Read the model definition and answer for the solid it produces. Units are mm, in the model's axes. A direction names the side the tool comes from. Coordinates: 2 decimals unless noted, no trailing zeros. Write each loop counter-clockwise with the first axis right and the second up, starting at its lowest first coordinate (ties: lowest second). Pieces come first, ordered by that corner, then holes. Notation, with made-up numbers: (59, -36.5) -> (69, -36.5) arc R28 cw to (69, -16.5) -> close; hole circle Ø7 at (42.25, 44.25). An arc over 180 degrees is marked (long way). Return JSON: item names as keys, results as strings.
from build123d import *

# Parameters (mm, degrees)
SKETCH1_R           = 2.286
SKETCH1_R_2         = 11.1125
BOSS_EXTRUDE1_DEPTH = 16.51
SKETCH2_R           = 12.7
CUT_EXTRUDE1_DEPTH  = 1.778
FILLET1_R           = 2.54


with BuildPart() as part:
    # Sketch1 → Boss-Extrude1 (new body)
    with BuildSketch(Plane(origin=(0, 0, 0), x_dir=(0, 0, -1), z_dir=(1, 0, 0))):
        with BuildLine():
            Line((-38.739778242, 0.742722084), (-14.609778242, -80.537277916))
            ThreePointArc((-14.609778242, -80.537277916), (3.522565818, -91.027310277), (14.999447267, -73.502930908))
            Line((14.999447267, -73.502930908), (6.35, -25.4))
            Line((6.35, -25.4), (6.35, 31.75))
            Line((6.35, 31.75), (-6.35, 31.75))
            Line((-6.35, 31.75), (-31.266140037, 18.54599812))
            ThreePointArc((-31.266140037, 18.54599812), (-38.182060342, 10.978915167), (-38.739778242, 0.742722084))
        make_face()
        Circle(SKETCH1_R, mode=Mode.SUBTRACT)
        with Locations((0, 25.4)):
            Circle(SKETCH1_R, mode=Mode.SUBTRACT)
        with Locations((0, -76.2)):
            Circle(SKETCH1_R_2, mode=Mode.SUBTRACT)
        with Locations((-24.13, 5.08)):
            Circle(SKETCH1_R_2, mode=Mode.SUBTRACT)
    extrude(amount=BOSS_EXTRUDE1_DEPTH)

    # Sketch2 → Cut-Extrude1 (cut)
    with BuildSketch(Plane(origin=(16.51, 0, 0), x_dir=(0, 0, -1), z_dir=(1, 0, 0))):
        with Locations((0, -76.2)):
            Circle(SKETCH2_R)
        with Locations((-24.13, 5.08)):
            Circle(SKETCH2_R)
    extrude(amount=-CUT_EXTRUDE1_DEPTH, mode=Mode.SUBTRACT)

    # Fillet1
    fillet1_edges = [part.edges().sort_by_distance(p)[0] for p in [
        (8.255, 31.75, 6.35),
        (8.255, 31.75, -6.35),
        (8.255, -25.4, -6.35),
    ]]
    fillet(fillet1_edges, radius=FILLET1_R)


solid = part.part
1. The part is cut by section D-D (z = 27). Determine the outline of the cut face in (x, y).
Taken from the geometry:
{"outline": "(0, -38.8) -> (16.51, -38.8) -> (16.51, -7.29) -> (14.73, -7.29) -> (14.73, -5.66) -> (0, -5.66) -> close; (0, 15.82) -> (14.73, 15.82) -> (14.73, 17.45) -> (16.51, 17.45) -> (16.51, 20.81) -> (0, 20.81) -> close"}
2. The part is cut by section B-B (y = 5.08). Determine the outline of the cut face in (x, z), then the cut area to 3 significant figures.
Taken from the geometry:
{"outline": "(0, -6.35) -> (16.51, -6.35) -> (16.51, 11.43) -> (14.73, 11.43) -> (14.73, 13.02) -> (0, 13.02) -> close; (0, 35.24) -> (14.73, 35.24) -> (14.73, 36.83) -> (16.51, 36.83) -> (16.51, 39.37) -> (0, 39.37) -> close", "area": "382 mm2"}
3. The part is cut by section A-A (z = 0). Determine the outline of the cut face in (x, y).
Taken from the geometry:
{"outline": "(0, -91.44) -> (16.51, -91.44) -> (16.51, -88.9) -> (14.73, -88.9) -> (14.73, -87.31) -> (0, -87.31) -> close; (0, -65.09) -> (14.73, -65.09) -> (14.73, -63.5) -> (16.51, -63.5) -> (16.51, -2.29) -> (0, -2.29) -> close; (0, 2.29) -> (16.51, 2.29) -> (16.51, 23.11) -> (0, 23.11) -> close; (0, 27.69) -> (16.51, 27.69) -> (16.51, 31.75) -> (0, 31.75) -> close"}
4. Consider L1, parallel to Y at x = 15.25, z = 0; L2, parallel to Y at x = 9.25, z = 0; L3, parallel to Z at x = 13, y = -86. Determine where each line is inside the solid, lowest interval first.
Taken from the geometry:
{"L1": "y = -91.44 to -88.9, -63.5 to -2.29, 2.29 to 23.11, 27.69 to 31.75", "L2": "y = -91.44 to -87.31, -65.09 to -2.29, 2.29 to 23.11, 27.69 to 31.75", "L3": "z = -11.67 to -5.24, 5.24 to 11.67"}
5. Flat-ended cylindrical pins translate along their axes: pin 1 Ø6 at (x, y) = (2.5, -6) entering from -Z; pin 2 Ø8 at (x, z) = (2.5, -9) entering from +Y; pin 3 Ø1.5 at (x, y) = (2.5, -65) entering from -Z; pin 4 Ø13.5 at (y, z) = (5.08, 24.13) entering from +X. Find the tip coordinate at first contact, or state that the pin passes through.
Taken from the geometry:
{"pin 1": "stops at z = -6.35", "pin 2": "stops at y = 31.45", "pin 3": "stops at z = -13.61", "pin 4": "passes through"}
6. A tool of negligible diameter and unlimited length cuts with its end or side. For faces 5 (the face through (14.732, -87.43, -0.88)), 6 (the face through (8.139, 11.114, 38.125)), 7 (the face through (8, 2, -6.35)), from which of +Z, -Z, +X, -X, +Y, -Y can it reach the whole face along a straight path? Write none if from no direction.
Taken from the geometry:
{"face 5": "+X", "face 6": "+Z, +X, -X", "face 7": "-Z, +X, -X, +Y"}
7. The part is cut by section C-C (x = 8). Count the separate pieces of the cut face and the enclosed holes in it, then the cut area to 3 significant figures.
Taken from the geometry:
{"separate pieces": "1", "enclosed holes": "4", "area": "3,490 mm2"}
8. For a pull along Z with two mould halves and no side action, classify faces 1 (the face through (8.371, 31.026, -5.586)), 2 (the face through (7.263, -66.83, -5.974)), 3 (the face through (8.14, -2.23, 0.5)), 4 (the face through (8, 31.75, 1)) as +Z half, -Z half, draft (parallel to the pull), parting line (faces both ways), or undercut.
Taken from the geometry:
{"face 1": "-Z half", "face 2": "undercut", "face 3": "undercut", "face 4": "draft"}
